```python
from build123d import *

# Parameters (mm, degrees)
F0_R     = 3.175
F1_DEPTH = 50.8
F2_SIZE  = 0.762
F3_R     = 1.5875
F4_DEPTH = 6.35


with BuildPart() as f1:
    # F0 (on Right) → F1 (new body)
    with BuildSketch(Plane.YZ):
        Circle(F0_R)
    extrude(amount=F1_DEPTH)

    # F2
    f2_edges = [f1.edges().sort_by_distance(p)[0] for p in [
        (25.4, 3.175, 0),
        (0, -3.175, 0),
        (50.8, -3.175, 0),
    ]]
    chamfer(f2_edges, length=F2_SIZE)


with BuildPart() as f4:
    # F3 (on Front) → F4 (new body, symmetric)
    with BuildSketch(Plane.XZ):
        with Locations((4.7625, 0)):
            Circle(F3_R)
    extrude(amount=F4_DEPTH, both=True)


with BuildPart() as f1_1:
    add(f1.part)

    # F5: cut F4
    add(f4.part, mode=Mode.SUBTRACT)


solid = f1_1.part
```
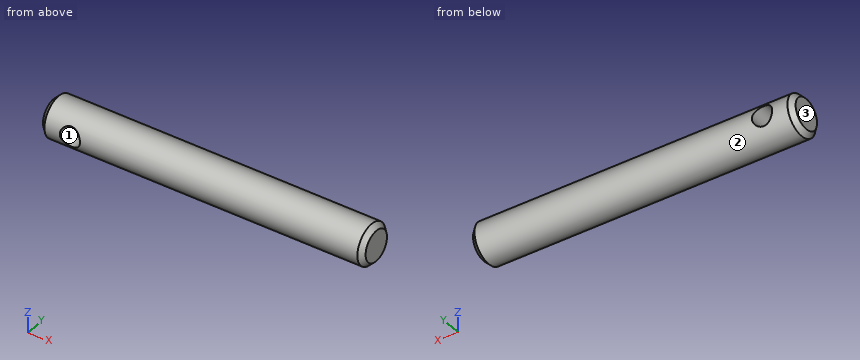
Here's how the part is built. I have some questions about the finished solid (model axes, mm). Face numbers are marked on the shaded views. Coordinates: 2 decimals unless noted, no trailing zeros. Order: outer loops, then holes, each group sorted by start corner. A loop starts at its lowest first (then second) coordinate and runs counter-clockwise, first axis right, second up. Notation, with made-up numbers: M -32.75,65 L -18.75,65 A7 cw -18.75,75 Z; hole C 36,38.25 d6. An arc over 180 degrees is marked long. Answer as a JSON object with one key per item and string values. Group by question number.
(1) I need wall thicknesses on probe 1 along X at (y, z) = (0, 0) (3 decimals); probe 2 along Y at (x, z) = (30.5, -0.25); probe 3 along Z at (x, y) = (3, -2.75). Which ranges of each line are inside material? Lowest first, please.
(2) Suppose I cut it at C-C, the plane x = 8. Please give me the cut outline in (y, z) (3 decimals), then the cut area to 3 significant figures.
(3) For pin 1 (1.5 mm diameter, centred on x = 39.5, z = 2, fed in from +Y); pin 2 (1 mm diameter, centred on x = 23.5, z = 1, fed in from +Y); pin 3 (2.5 mm diameter, centred on x = 4.76, z = 0, fed in from +Y), each with a flat end and sliding along its axis, tell me the tip position at first contact or that it passes through.
(4) Suppose I cut it at A-A, the plane z = 0. Please give me the cut outline in (x, y) (3 decimals), then the cut area to 3 significant figures.
(5) If we mould it in two halves opening along Z, with no side actions, what happens to the marked faces 1, 2 and 3? For each: released by +Z, released by -Z, zero draft, split by the parting line, or undercut.
Values found:
{
 "1": {"probe 1": "x = 0 to 3.175, 6.35 to 50.8", "probe 2": "y = -3.17 to 3.17", "probe 3": "z = -1.59 to 1.59"},
 "2": {"outline": "C 0,0 d6.35", "area": "31.7 mm^2"},
 "3": {"pin 1": "stops at y = 2.92", "pin 2": "stops at y = 3.14", "pin 3": "passes through"},
 "4": {"outline": "M 0,-2.413 L 0.762,-3.175 L 3.175,-3.175 L 3.175,3.175 L 0.762,3.175 L 0,2.413 Z; M 6.35,-3.175 L 50.038,-3.175 L 50.8,-2.413 L 50.8,2.413 L 50.038,3.175 L 6.35,3.175 Z", "area": "301 mm^2"},
 "5": {"face 1": "undercut", "face 2": "split by the parting line", "face 3": "zero draft"}
}
